```python
from build123d import *

# Parameters (mm, degrees)
F0_W     = 950
F0_H     = 350
F1_DEPTH = 900
F2_T     = -50
F3_W     = 950
F3_H     = 350
F4_DEPTH = 79.1636947542
F5_T     = -10


with BuildPart() as f1:
    # F0 (on Top) → F1 (new body)
    with BuildSketch(Plane.XY):
        Rectangle(F0_W, F0_H)
    extrude(amount=F1_DEPTH)

    # F2
    f2_openings = [f1.faces().sort_by_distance(p)[0] for p in [
        (0, -175, 450),
        (0, 0, 0),
        (0, 175, 450),
    ]]
    offset(amount=F2_T, openings=f2_openings)

    # F3 (on face) → F4 (join)
    with BuildSketch(Plane.XY.offset(900)):
        Rectangle(F3_W, F3_H)
    extrude(amount=F4_DEPTH)

    # F5
    f5_openings = [f1.faces().sort_by_distance(p)[0] for p in [
        (-450, -175, 13.642806),
    ]]
    offset(amount=F5_T, openings=f5_openings, kind=Kind.INTERSECTION)


solid = f1.part
```
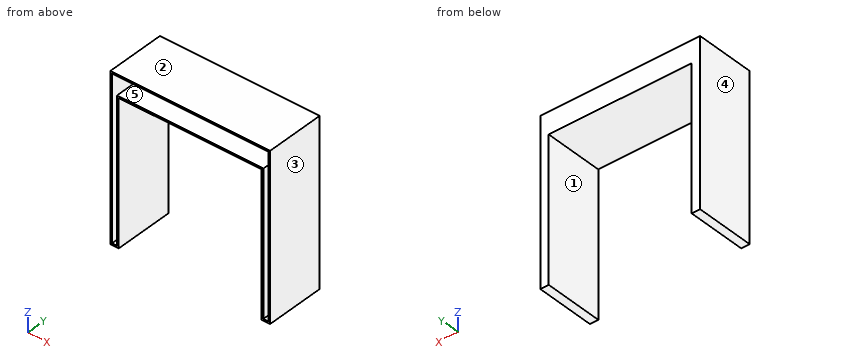
For this review, take the finished solid that the model builds, in its own axes (mm). Face numbers are marked on the shaded views. A direction names the side the tool comes from. Give positions to 0.01 mm unless a question says otherwise; leave off trailing zeros. Order: outer loops, then holes, each group sorted by start corner. A loop starts at its lowest first (then second) coordinate and runs counter-clockwise, first axis right, second up.
1) Take a section at C-C (y = -53). Give the boundary of the cut face in (x, z), then the cut area to 3 significant figures.
2) The part is to be moulded in two halves that separate along X. For the marked faces 3, 4 and 5, say which applies: released by +X, released by -X, zero draft, split by the parting line, or undercut.
3) Wall thickness on line 1 (X direction, y = -115, z = 147); line 2 (Z direction, x = -261, y = 10.5); line 3 (X direction, y = -102.5, z = 894): over which ranges is each line inside the solid? List them lowest first.
4) Take a section at A-A (z = 172.5). Give the boundary of the cut face in (x, y), then the cut area to 3 significant figures.
5) For the marked faces 1 and 2, list the 3-axis set-ups (+Z, -Z, +X, -X, +Y, -Y) from which the entire face can be reached by the end or side of a thin tool; tool diameter is ignored.
6) Take a section at B-B (x = -365). Give the boundary of the cut face in (y, z), then the cut area to 3 significant figures.
Derived:
1. outline: (-475, 0) - (-425, 0) - (-425, 850) - (425, 850) - (425, 0) - (475, 0) - (475, 979.16) - (-475, 979.16) - close; hole (-465, 10) - (-435, 10) - (-435, 860) - (435, 860) - (435, 10) - (465, 10) - (465, 969.16) - (-465, 969.16) - close
1. area: 55,200 mm2
2. face 3: released by +X
2. face 4: released by -X
2. face 5: undercut
3. line 1: x = -475 to -465, -435 to -425, 425 to 435, 465 to 475
3. line 2: z = 850 to 860, 969.16 to 979.16
3. line 3: x = -475 to -465, 465 to 475
4. outline: (-475, -175) - (-465, -175) - (-465, 165) - (-435, 165) - (-435, -175) - (-425, -175) - (-425, 175) - (-475, 175) - close; (425, -175) - (435, -175) - (435, 165) - (465, 165) - (465, -175) - (475, -175) - (475, 175) - (425, 175) - close
4. area: 14,600 mm2
5. face 1: -Z, +Y, -Y
5. face 2: +Z, +X, -X, +Y, -Y
6. outline: (-175, 850) - (175, 850) - (175, 979.16) - (-175, 979.16) - (-175, 969.16) - (165, 969.16) - (165, 860) - (-175, 860) - close
6. area: 8,090 mm2
